For this review, take the finished solid that the model builds, in its own axes (mm). A direction names the side the tool comes from. Give positions to 0.01 mm unless a question says otherwise; leave off trailing zeros. Write each loop counter-clockwise with the first axis right and the second up, starting at its lowest first coordinate (ties: lowest second). Pieces come first, ordered by that corner, then holes. Notation, with made-up numbers: M 2,56.5 L 35,56.5 A16 ccw 35,85.5 Z; hole C -7,40 d1. An arc over 180 degrees is marked long. One line per item, written item: value. Start each with the question number.
Item 1: Mouldability with a two-part tool opening along X and no side actions: class faces 4 (the face through (0, 0, 14.25)), 5 (the face through (-1.73, -7.81, 25.64)), 6 (the face through (-4, 2, 52)) as released by +X, released by -X, zero draft, split by the parting line, or undercut.
Item 2: Consider section C-C, the plane z = 44. Write out the cut boundary in (x, y).
Item 3: Clearance check with flat-ended pins moving along their axes: pin 1 Ø1.5 at (x, z) = (-3, 8.5) entering from +Y; pin 2 Ø2.5 at (x, y) = (-0.5, 0.5) entering from +Z; pin 3 Ø1 at (y, z) = (-6, 14.5) entering from +X. State where each tip first meets the part, or that it passes through.
Item 4: Consider section A-A, the plane y = 0. Write out the cut boundary in (x, z).
Item 5: To check wall thickness, follow probe 1 along Y at (x, z) = (0, 8.25); probe 2 along Z at (x, y) = (-2.5, 1.5); probe 3 along Y at (x, z) = (-2.25, 41). State the ranges of each line that lie inside material, in increasing order.
Item 6: Consider section D-D, the plane z = 21. Write out the cut boundary in (x, y).
Item 7: Tool access review of faces 1 (the face through (-0.878, -3.954, 44.775)), 2 (the face through (-0.878, -3.954, 7.025)), 3 (the face through (-4, 2, 0)): name each direction out of +Z, -Z, +X, -X, +Y, -Y from which nothing blocks a thin tool from reaching the whole face with its end or side.
```python
from build123d import *

# Parameters (mm, degrees)
S01_SOLID_POST_BLANK_16_MM_R             = 8
F_01_SOLID_POST_BLANK_16_MM_DEPTH        = 52
F_02_START                               = -0.1
S02_REAR_M6_HEAT_SET_INSERT_SEAT_R       = 4.05
F_02_REAR_M6_HEAT_SET_INSERT_SEAT_DEPTH  = 14.35
F_03_START                               = 37.75
S03_FRONT_M6_HEAT_SET_INSERT_SEAT_R      = 4.05
F_03_FRONT_M6_HEAT_SET_INSERT_SEAT_DEPTH = 14.35


with BuildPart() as part:
    # S01 - Solid post blank - 16 mm → 01 - Solid post blank - 16 mm (new body)
    with BuildSketch(Plane.XY):
        Circle(S01_SOLID_POST_BLANK_16_MM_R)
    extrude(amount=F_01_SOLID_POST_BLANK_16_MM_DEPTH)

    # S02 - Rear M6 heat-set insert seat → 02 - Rear M6 heat-set insert seat (cut)
    with BuildSketch(Plane.XY.offset(F_02_START)):
        Circle(S02_REAR_M6_HEAT_SET_INSERT_SEAT_R)
    extrude(amount=F_02_REAR_M6_HEAT_SET_INSERT_SEAT_DEPTH, mode=Mode.SUBTRACT)

    # S03 - Front M6 heat-set insert seat → 03 - Front M6 heat-set insert seat (cut)
    with BuildSketch(Plane.XY.offset(F_03_START)):
        Circle(S03_FRONT_M6_HEAT_SET_INSERT_SEAT_R)
    extrude(amount=F_03_FRONT_M6_HEAT_SET_INSERT_SEAT_DEPTH, mode=Mode.SUBTRACT)


solid = part.part
```
Model answer:
1. face 4: undercut
1. face 5: split by the parting line
1. face 6: zero draft
2. outline: C 0,0 d16; hole C 0,0 d8.1
3. pin 1: stops at y = 7.68
3. pin 2: stops at z = 37.75
3. pin 3: stops at x = 5.81
4. outline: M -8,0 L -4.05,0 L -4.05,14.25 L 4.05,14.25 L 4.05,0 L 8,0 L 8,52 L 4.05,52 L 4.05,37.75 L -4.05,37.75 L -4.05,52 L -8,52 Z
5. probe 1: y = -8 to -4.05, 4.05 to 8
5. probe 2: z = 14.25 to 37.75
5. probe 3: y = -7.68 to -3.37, 3.37 to 7.68
6. outline: C 0,0 d16
7. face 1: +Z
7. face 2: -Z
7. face 3: -Z, +X, -X, +Y, -Y
